Input: part model. Units: mm. Frame: model coordinates. A direction names the side the tool comes from. Round coordinates to 2 decimals unless told otherwise and drop trailing zeros. Loops run counter-clockwise (first coordinate to the right, second up) from the corner with the lowest first, then second, coordinate; pieces in that order, holes last. Notation, with made-up numbers: M -8,68 L 13,68 A12 ccw 13,91 Z; hole C 19,85.5 d6. An arc over 180 degrees is marked long. Return JSON: item names as keys, results as strings. Group by question number.
1) Access query for faces 1 (the face through (-2.74, -2.1, 2.54)), 2 (the face through (3, 2, 10)), 3 (the face through (2, -4, 5)). Directions: +Z, -Z, +X, -X, +Y, -Y. A direction counts if a zero-diameter tool reaches every point of the face in a straight line with its end or side. Return the directions, or none.
2) Mould query, pull axis X, two halves, no side actions, for faces 4 (the face through (-3.624, -2.545, 7.465)), 5 (the face through (0, -4, 0)), 6 (the face through (0.8, -3.1, 5)). Classes: +X half, -X half, draft (parallel to the pull), parting line (faces both ways), or undercut.
3) Section B-B (x = -2.75). Output: boundary loops of the cut face in (y, z), plus the area to 3 significant figures.
4) Material intervals for line 1 (X direction, y = 2.75, z = 0.75); line 2 (Z direction, x = 5.25, y = 1.25); line 3 (Y direction, x = -1, z = 7.75), sorted ascending. Write a range as from..to.
5) Section A-A (y = -1). Output: boundary loops of the cut face in (x, z), plus the area to 3 significant figures.
6) Section D-D (y = -4). Output: boundary loops of the cut face in (x, z).
7) Contact query for flat-ended pins moving along their axis: P1, Ø4, axis at x = -4.5, z = 1, coming from the +Y side; P2, Ø2, axis at x = 3, y = 2.5, coming from the -Z side; P3, Ø3, axis at y = -5, z = 5, coming from the +X side; P4, Ø3.5, axis at x = 1.5, y = 0.5, coming from the -Z side. Output: stop coordinate, or through.
8) Section C-C (z = 2). Output: boundary loops of the cut face in (x, y).
from build123d import *

# Parameters (mm, degrees)
SKETCH1_R           = 10
BOSS_EXTRUDE2_DEPTH = 5
SKETCH2_R           = 4.5
SKETCH2_R_2         = 3.25
BOSS_EXTRUDE3_DEPTH = 5
SKETCH3_R           = 3.450600028
CUT_EXTRUDE1_DEPTH  = 5


with BuildPart() as part:
    # Sketch1 → Boss-Extrude2 (new body)
    with BuildSketch(Plane.XY):
        Circle(SKETCH1_R)
    extrude(amount=BOSS_EXTRUDE2_DEPTH)

    # Sketch2 → Boss-Extrude3 (add)
    with BuildSketch(Plane.XY.offset(5)):
        with Locations((-0.053141413, 0.193433093)):
            Circle(SKETCH2_R)
        with Locations((-0.053141413, 0.193433093)):
            Circle(SKETCH2_R_2, mode=Mode.SUBTRACT)
    extrude(amount=BOSS_EXTRUDE3_DEPTH)

    # Sketch3 → Cut-Extrude1 (cut)
    with BuildSketch(Plane.XY.offset(5)):
        Circle(SKETCH3_R)
    extrude(amount=-CUT_EXTRUDE1_DEPTH, mode=Mode.SUBTRACT)


solid = part.part
Returned:
{
 "1": {"face 1": "-Z", "face 2": "+Z, +X, -X, +Y, -Y", "face 3": "+Z"},
 "2": {"face 4": "parting line", "face 5": "draft", "face 6": "undercut"},
 "3": {"outline": "M -9.61,0 L -2.08,0 L -2.08,5 L -1.62,5 L -1.62,10 L -3.41,10 L -3.41,5 L -9.61,5 Z; M 2.01,5 L 2.08,5 L 2.08,0 L 9.61,0 L 9.61,5 L 3.8,5 L 3.8,10 L 2.01,10 Z", "area": "93.2 mm^2"},
 "4": {"line 1": "x = -9.61..-2.08, 2.08..9.61", "line 2": "z = 0..5", "line 3": "y = -4.21..-2.92, 3.3..4.59"},
 "5": {"outline": "M -9.95,0 L -3.3,0 L -3.3,5 L -3.08,5 L -3.08,10 L -4.39,10 L -4.39,5 L -9.95,5 Z; M 2.97,5 L 3.3,5 L 3.3,0 L 9.95,0 L 9.95,5 L 4.29,5 L 4.29,10 L 2.97,10 Z", "area": "79.6 mm^2"},
 "6": {"outline": "M -9.17,0 L 9.17,0 L 9.17,5 L 1.58,5 L 1.58,10 L -1.69,10 L -1.69,5 L -9.17,5 Z"},
 "7": {"P1": "stops at y = 9.68", "P2": "stops at z = 0", "P3": "stops at x = 9.37", "P4": "stops at z = 5"},
 "8": {"outline": "C 0,0 d20; hole C 0,0 d6.9"}
}
